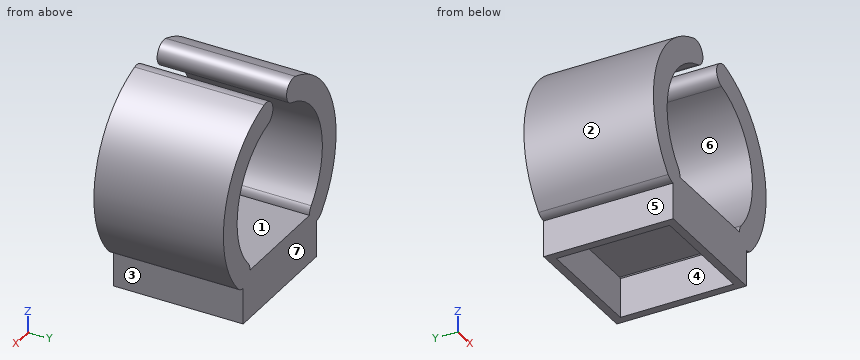
from build123d import *

# Parameters (mm, degrees)
F0_W     = 16
F0_H     = 16
F1_DEPTH = 6
F2_T     = -1
F4_DEPTH = 16


with BuildPart() as f1:
    # F0 (on Top) → F1 (new body)
    with BuildSketch(Plane.XY):
        with Locations((8, -8)):
            Rectangle(F0_W, F0_H)
    extrude(amount=F1_DEPTH)

    # F2
    f2_openings = [f1.faces().sort_by_distance(p)[0] for p in [
        (8, -8, 0),
    ]]
    offset(amount=F2_T, openings=f2_openings)

    # F3 (on Front) → F4 (join)
    with BuildSketch(Plane.XZ):
        with BuildLine():
            ThreePointArc((14.891778, 7.010863), (14.989137, 4.891778), (17.108222, 4.989137))
            ThreePointArc((17.108222, 4.989137), (19.863955, 16.648312), (11.415583, 25.142748))
            ThreePointArc((11.415583, 25.142748), (9.558719, 24.11705), (10.584417, 22.260186))
            ThreePointArc((10.584417, 22.260186), (16.976916, 15.832832), (14.891778, 7.010863))
        make_face()
        with BuildLine():
            ThreePointArc((4.584417, 25.142748), (-3.863955, 16.648312), (-1.108222, 4.989137))
            ThreePointArc((-1.108222, 4.989137), (1.010863, 4.891778), (1.108222, 7.010863))
            ThreePointArc((1.108222, 7.010863), (-0.976916, 15.832832), (5.415583, 22.260186))
            ThreePointArc((5.415583, 22.260186), (6.441281, 24.11705), (4.584417, 25.142748))
        make_face()
    extrude(amount=F4_DEPTH)


solid = f1.part
Design review of the part built by this model. Coordinates are the model's own, in mm. Face numbers are marked on the shaded views. A direction names the side the tool comes from. Coordinates: 2 decimals unless noted, no trailing zeros. Order: outer loops, then holes, each group sorted by start corner. A loop starts at its lowest first (then second) coordinate and runs counter-clockwise, first axis right, second up. Notation, with made-up numbers: (57.5, -17) -> (89.5, -17) arc R13 ccw to (89.5, -13) -> close; hole circle Ø9 at (50, 10.25). An arc over 180 degrees is marked (long way). Use one line per item in the form item = value. Start each with the question number.
(1) Add section C-C on y = -7.25. State the section outline as (x, z) points, plus the area to 3 significant figures.
(2) For probe 1 along Y at (x, z) = (13.5, 2.5); probe 2 along X at (y, z) = (-3.75, 13); probe 3 along X at (y, z) = (-2.75, 21), list the stretches that pass through material, from the lowest coordinate up.
(3) Insertion check: pin 1 (8 mm diameter, centred on y = -10, z = 4.5, fed in from -X); pin 2 (1.3 mm diameter, centred on y = -6.5, z = 3, fed in from -X); pin 3 (2.5 mm diameter, centred on x = 6.5, z = 2, fed in from +Y); pin 4 (5.5 mm diameter, centred on y = -9.5, z = 3, fed in from +X). Each pin has a flat end and moves straight along its axis. Give the tip position at first contact, or say it passes through.
(4) For the marked faces 4, 5, 6 and 7, list the 3-axis set-ups (+Z, -Z, +X, -X, +Y, -Y) from which the entire face can be reached by the end or side of a thin tool; tool diameter is ignored.
(5) The part is to be moulded in two halves that separate along X. For the marked faces 1, 2 and 3, say which applies: +X half, -X half, draft (parallel to the pull), parting line (faces both ways), or undercut.
(6) Add section B-B on z = 15.75. State the section outline as (x, y) points, plus the area to 3 significant figures.
(7) Add section D-D on z = 9.25. State the section outline as (x, y) points.
(8) Add section A-A on x = 5. State the section outline as (y, z) points, plus the area to 3 significant figures.
Answer block:
q1.outline = (-1.11, 4.99) arc R1.5 ccw to (0, 4.5) -> (0, 0) -> (1, 0) -> (1, 4.88) arc R1.5 ccw to (1.12, 5) -> (14.88, 5) arc R1.5 ccw to (15, 4.88) -> (15, 0) -> (16, 0) -> (16, 4.5) arc R1.5 ccw to (17.11, 4.99) arc R12.33 ccw to (11.42, 25.14) arc R1.5 ccw to (10.58, 22.26) arc R9.33 cw to (14.89, 7.01) arc R1.5 ccw to (14.5, 6) -> (1.5, 6) arc R1.5 ccw to (1.11, 7.01) arc R9.33 cw to (5.42, 22.26) arc R1.5 ccw to (4.58, 25.14) arc R12.33 ccw to start
q1.area = 168 mm²
q2.probe_1 = -16 to -15, -1 to 0
q2.probe_2 = -4.32 to -1.32, 17.32 to 20.32
q2.probe_3 = -1.63 to 2.74, 13.26 to 17.63
q3.pin_1 = -3.36
q3.pin_2 = 0
q3.pin_3 = 0
q3.pin_4 = 17.75
q4.face_4 = -Z
q4.face_5 = -Z, -X, +Y, -Y
q4.face_6 = +Y, -Y
q4.face_7 = +Z, -Z, +X, -X, +Y
q5.face_1 = undercut
q5.face_2 = -X half
q5.face_3 = +X half
q6.outline = (-4.08, -16) -> (-1, -16) -> (-1, 0) -> (-4.08, 0) -> close; (17, -16) -> (20.08, -16) -> (20.08, 0) -> (17, 0) -> close
q6.area = 98.6 mm²
q7.outline = (-3.64, -16) -> (-0.4, -16) -> (-0.4, 0) -> (-3.64, 0) -> close; (16.4, -16) -> (19.64, -16) -> (19.64, 0) -> (16.4, 0) -> close
q8.outline = (-16, 0) -> (-15, 0) -> (-15, 5) -> (-1, 5) -> (-1, 0) -> (0, 0) -> (0, 6) -> (-16, 6) -> close; (-16, 22.13) -> (0, 22.13) -> (0, 25.2) -> (-16, 25.2) -> close
q8.area = 75.1 mm²
